Design review of the part built by this model. Coordinates are the model's own, in mm. Face numbers are marked on the shaded views. Round coordinates to 2 decimals unless told otherwise and drop trailing zeros. Write each loop counter-clockwise with the first axis right and the second up, starting at its lowest first coordinate (ties: lowest second). Pieces come first, ordered by that corner, then holes. Notation, with made-up numbers: (55, 60) -> (102, 60) arc R16 ccw to (102, 73) -> close; hole circle Ø6 at (3.5, 74). An arc over 180 degrees is marked (long way). One line per question, with ' | ' between items. Start each with the question number.
1) Insertion check: pin 1 Ø3.5 at (x, z) = (10, 0) entering from +Y. The pin has a flat end and moves straight along its axis. Give the tip position at first contact, or say it passes through.
2) For probe 1 along Z at (x, y) = (10, 13.65); probe 2 along Y at (x, z) = (10.5, -0.25); probe 3 along X at (y, z) = (14, 0.9), list the stretches that pass through material, from the lowest coordinate up.
3) Consider section C-C (z = 0). Give the boundary of the cut face in (x, y), then the cut area to 4 significant figures.
4) Mouldability with a two-part tool opening along X and no side actions: class the marked faces 1, 2, 3 and 4 as +X half, -X half, draft (parallel to the pull), parting line (faces both ways), or undercut.
5) Consider section B-B (x = -10). Give the boundary of the cut face in (y, z).
6) Consider section A-A (y = 12.25). Give the boundary of the cut face in (x, z), then the cut area to 3 significant figures.
```python
from build123d import *

# Parameters (mm, degrees)
F0_W     = 30
F0_H     = 6
F1_DEPTH = 15
F2_R     = 2.1
F3_DEPTH = 5
F4_SIZE  = 0.5


with BuildPart() as f1:
    # F0 (on Front) → F1 (new body)
    with BuildSketch(Plane.XZ):
        Rectangle(F0_W, F0_H)
    extrude(amount=-F1_DEPTH)

    # F2 (on face) → F3 (cut)
    with BuildSketch(Plane(origin=(0, 15, 0), x_dir=(-1, 0, 0), z_dir=(0, 1, 0))):
        with Locations((-10, 0)):
            Circle(F2_R)
        with Locations((10, 0)):
            Circle(F2_R)
    extrude(amount=-F3_DEPTH, mode=Mode.SUBTRACT)

    # F4
    f4_edges = [f1.edges().sort_by_distance(p)[0] for p in [
        (15, 7.5, 3),
        (-15, 7.5, 3),
        (0, 0, 3),
        (0, 15, 3),
        (-15, 7.5, -3),
        (15, 7.5, -3),
        (0, 0, -3),
        (0, 15, -3),
        (15, 0, 0),
        (15, 15, 0),
        (-15, 0, 0),
        (-15, 15, 0),
    ]]
    chamfer(f4_edges, length=F4_SIZE)


solid = f1.part
```
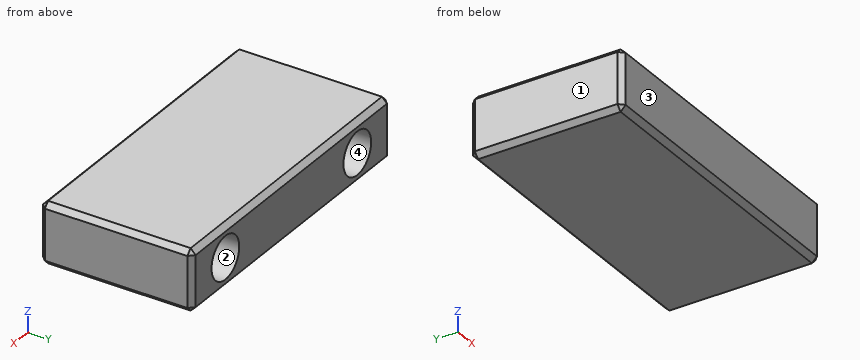
From the geometry:
1) pin 1: stops at y = 10
2) probe 1: z = -3 to -2.1, 2.1 to 3 | probe 2: y = 0 to 10 | probe 3: x = -15 to -11.9, -8.1 to 8.1, 11.9 to 15
3) outline: (-15, 0.5) -> (-14.5, 0) -> (14.5, 0) -> (15, 0.5) -> (15, 14.5) -> (14.5, 15) -> (12.1, 15) -> (12.1, 10) -> (7.9, 10) -> (7.9, 15) -> (-7.9, 15) -> (-7.9, 10) -> (-12.1, 10) -> (-12.1, 15) -> (-14.5, 15) -> (-15, 14.5) -> close | area: 407.5 mm2
4) face 1: -X half | face 2: undercut | face 3: draft | face 4: undercut
5) outline: (0, -2.5) -> (0.5, -3) -> (14.5, -3) -> (15, -2.5) -> (15, -2.1) -> (10, -2.1) -> (10, 2.1) -> (15, 2.1) -> (15, 2.5) -> (14.5, 3) -> (0.5, 3) -> (0, 2.5) -> close
6) outline: (-15, -2.5) -> (-14.5, -3) -> (14.5, -3) -> (15, -2.5) -> (15, 2.5) -> (14.5, 3) -> (-14.5, 3) -> (-15, 2.5) -> close; hole circle Ø4.2 at (-10, 0); hole circle Ø4.2 at (10, 0) | area: 152 mm2
